from build123d import *

# Parameters (mm, degrees)
F0_R     = 33.613844165
F0_R_2   = 7.3530240303
F1_DEPTH = 12.7
F2_DEPTH = 25.4


with BuildPart() as f1:
    # F0 (on Front) → F1 (new body)
    with BuildSketch(Plane.XZ):
        Circle(F0_R)
        with BuildLine():
            ThreePointArc((4.7208512746, -19.951569966), (4.6925332266, -19.9590350044), (4.6642082743, -19.9664738029))
            ThreePointArc((4.6642082743, -19.9664738029), (4.6934800842, -19.9547063806), (4.7227373879, -19.9429029377))
            ThreePointArc((4.7227373879, -19.9429029377), (4.7217944882, -19.947236486), (4.7208512746, -19.951569966))
        make_face(mode=Mode.SUBTRACT)
        Circle(F0_R_2, mode=Mode.SUBTRACT)
        with BuildLine():
            ThreePointArc((14.5159144375, 14.0511614861), (14.5316083012, 14.029833317), (14.547274448, 14.0084847808))
            ThreePointArc((14.547274448, 14.0084847808), (14.5285756501, 14.0288524457), (14.5098472673, 14.0491929102))
            ThreePointArc((14.5098472673, 14.0491929102), (14.5128808291, 14.0501772698), (14.5159144375, 14.0511614861))
        make_face(mode=Mode.SUBTRACT)
        Circle(F0_R_2)
    extrude(amount=F1_DEPTH)

    # F0 (on Front) → F2 (join)
    with BuildSketch(Plane.XZ):
        Circle(F0_R)
        with BuildLine():
            ThreePointArc((4.7208512746, -19.951569966), (4.6925332266, -19.9590350044), (4.6642082743, -19.9664738029))
            ThreePointArc((4.6642082743, -19.9664738029), (4.6934800842, -19.9547063806), (4.7227373879, -19.9429029377))
            ThreePointArc((4.7227373879, -19.9429029377), (4.7217944882, -19.947236486), (4.7208512746, -19.951569966))
        make_face(mode=Mode.SUBTRACT)
        Circle(F0_R_2, mode=Mode.SUBTRACT)
        with BuildLine():
            ThreePointArc((14.5159144375, 14.0511614861), (14.5316083012, 14.029833317), (14.547274448, 14.0084847808))
            ThreePointArc((14.547274448, 14.0084847808), (14.5285756501, 14.0288524457), (14.5098472673, 14.0491929102))
            ThreePointArc((14.5098472673, 14.0491929102), (14.5128808291, 14.0501772698), (14.5159144375, 14.0511614861))
        make_face(mode=Mode.SUBTRACT)
    extrude(amount=F2_DEPTH)


solid = f1.part
Work out the finished part from the listing and answer in its coordinate system (mm). A direction names the side the tool comes from. Coordinates: 2 decimals unless noted, no trailing zeros. Write each loop counter-clockwise with the first axis right and the second up, starting at its lowest first coordinate (ties: lowest second). Pieces come first, ordered by that corner, then holes. Notation, with made-up numbers: M -13,41 L 32,41 A17 cw 32,72 Z; hole C 15,31 d11. An arc over 180 degrees is marked long. Write item = value, one per line.
1. For faces 1 (the face through (0, -12.7, 0)), 2 (the face through (-8, -25.4, 0)), determine the directions among +Z, -Z, +X, -X, +Y, -Y from which every point of the face is accessible in a straight line to the end or side of a thin tool.
Solution:
face_1 = -Y
face_2 = +Z, -Z, +X, -X, -Y
2. Straight lines are drawn through the part: line 1 (Z direction, x = 0, y = -21.5); line 2 (Z direction, x = 0.5, y = -15.25); line 3 (X direction, y = -10, z = -1). For each, find the intervals that lie inside material, in ascending order. Write a range as from..to.
Solution:
line_1 = -33.61..-7.35, 7.35..33.61
line_2 = -33.61..-7.34, 7.34..33.61
line_3 = -33.6..33.6
3. The part is cut by section C-C (z = 0). Determine the outline of the cut face in (x, y).
Solution:
outline = M -33.61,-25.4 L -7.35,-25.4 L -7.35,-12.7 L 7.35,-12.7 L 7.35,-25.4 L 33.61,-25.4 L 33.61,0 L -33.61,0 Z
4. The part is cut by section D-D (x = 0). Determine the outline of the cut face in (y, z).
Solution:
outline = M -25.4,-33.61 L 0,-33.61 L 0,33.61 L -25.4,33.61 L -25.4,7.35 L -12.7,7.35 L -12.7,-7.35 L -25.4,-7.35 Z
5. Flat-ended cylindrical pins translate along their axes: pin 1 (7.5 mm diameter, centred on x = -2.5, z = -2.5, fed in from -Y); pin 2 (2 mm diameter, centred on y = -4, z = 10.5, fed in from -X); pin 3 (2 mm diameter, centred on x = 12, y = -17.5, fed in from +Z). Find the tip coordinate at first contact, or state that the pin passes through.
Solution:
pin_1 = -12.7
pin_2 = -32.24
pin_3 = 31.76
